```python
from build123d import *

# Parameters (mm, degrees)
BOSS_EXTRUDE1_DEPTH = 0.4
CUT_EXTRUDE1_REACH  = 2.4
SKETCH2_R           = 0.75
FILLET1_R           = 0.5
FILLET2_R           = 0.7
FILLET3_R           = 1.1


with BuildPart() as part:
    # Sketch1 → Boss-Extrude1 (new body)
    with BuildSketch(Plane.XY):
        with BuildLine():
            Line((11.400711478, -0.747727009), (10.812582712, 0.284))
            Line((10.812582712, 0.284), (9.577065579, 0.284))
            ThreePointArc((9.577065579, 0.284), (8.441, 0.429), (7.304934421, 0.284))
            Line((7.304934421, 0.284), (1.421915609, 0.284))
            ThreePointArc((1.421915609, 0.284), (-1.127957488, 0.911159648), (0.021323855, -1.449843196))
            Line((0.021323855, -1.449843196), (0.658996505, -1.291597308))
            ThreePointArc((0.658996505, -1.291597308), (2.462224804, -1.094137246), (4.253267655, -1.381866782))
            ThreePointArc((4.253267655, -1.381866782), (5.15625108, -0.593183537), (6.321, -0.309))
            Line((6.321, -0.309), (7.350233295, -0.309))
            ThreePointArc((7.350233295, -0.309), (8.381, -0.429), (9.411766705, -0.309))
            Line((9.411766705, -0.309), (10.075524156, -0.309))
            Line((10.075524156, -0.309), (10.589288522, -1.210272991))
            ThreePointArc((10.589288522, -1.210272991), (11.226272991, -1.384711478), (11.400711478, -0.747727009))
        make_face()
    extrude(amount=BOSS_EXTRUDE1_DEPTH)

    # Sketch2 → Cut-Extrude1 (cut, up to next)
    with BuildSketch(Plane.XY, mode=Mode.PRIVATE) as cut_extrude1_sk1:
        Circle(SKETCH2_R)
    cut_extrude1_tool1 = extrude(cut_extrude1_sk1.sketch, amount=CUT_EXTRUDE1_REACH, mode=Mode.PRIVATE) & part.part
    add(cut_extrude1_tool1.solids().sort_by_distance((0, 0, 0))[0], mode=Mode.SUBTRACT)

    # Fillet1
    fillet1_edges = [part.edges().sort_by_distance(p)[0] for p in [
        (10.075524156, -0.309, 0.2),
    ]]
    fillet(fillet1_edges, radius=FILLET1_R)

    # Fillet2
    fillet2_edges = [part.edges().sort_by_distance(p)[0] for p in [
        (1.421915609, 0.284, 0.2),
    ]]
    fillet(fillet2_edges, radius=FILLET2_R)

    # Fillet3
    fillet3_edges = [part.edges().sort_by_distance(p)[0] for p in [
        (0.021323855, -1.449843196, 0.2),
        (4.253267655, -1.381866782, 0.2),
    ]]
    fillet(fillet3_edges, radius=FILLET3_R)


solid = part.part
```
The model under review builds one solid part; all positions refer to its coordinate system, in mm. Round coordinates to 2 decimals unless told otherwise and drop trailing zeros. Order: outer loops, then holes, each group sorted by start corner. A loop starts at its lowest first (then second) coordinate and runs counter-clockwise, first axis right, second up.
Item 1: For pin 1 (1 mm diameter, centred on x = 8, y = -1, fed in from +Z), flat-tipped, find the tip position at first contact; note if it passes through.
Working result:
pin 1: passes through
Item 2: Add section C-C, the plane y = 1.05. State the section outline as (x, z) points.
Working result:
outline: (-1, 0) - (1, 0) - (1, 0.4) - (-1, 0.4) - close
Item 3: Add section D-D, the plane x = 5.75. State the section outline as (y, z) points.
Working result:
outline: (-0.37, 0) - (0.28, 0) - (0.28, 0.4) - (-0.37, 0.4) - close
Item 4: To check wall thickness, follow probe 1 along Y at (x, z) = (0, 0.1); probe 2 along X at (y, z) = (0.05, 0.2); probe 3 along X at (y, z) = (-1, 0.35). State the ranges of each line that lie inside material, in increasing order.
Working result:
probe 1: y = -1.44 to -0.75, 0.75 to 1.45
probe 2: x = -1.45 to -0.75, 0.75 to 10.95
probe 3: x = -1.05 to 4.58, 10.47 to 11.46
Item 5: Draft analysis for pull direction Y (two halves, no side actions). For faces 1 (the cylindrical face through (-1.12, 0.92, 0.2)), 2 (the flat face through (3, 0, 0)), 3 (the cylindrical face through (-0.75, 0.03, 0.2)), state which applies: released by +Y, released by -Y, zero draft, split by the parting line, or undercut.
Working result:
face 1: split by the parting line
face 2: zero draft
face 3: undercut
Item 6: Add section B-B, the plane x = 0. State the section outline as (y, z) points.
Working result:
outline: (-1.44, 0) - (-0.75, 0) - (-0.75, 0.4) - (-1.44, 0.4) - close; (0.75, 0) - (1.45, 0) - (1.45, 0.4) - (0.75, 0.4) - close
Item 7: Add section A-A, the plane y = 0. State the section outline as (x, z) points, and give its area (3 significant figures).
Working result:
outline: (-1.45, 0) - (-0.75, 0) - (-0.75, 0.4) - (-1.45, 0.4) - close; (0.75, 0) - (10.97, 0) - (10.97, 0.4) - (0.75, 0.4) - close
area: 4.37 mm2
